The listing builds one solid part. Answer for the finished solid, in the listing's coordinates (mm). A direction names the side the tool comes from. Round coordinates to 2 decimals unless told otherwise and drop trailing zeros. Loops run counter-clockwise (first coordinate to the right, second up) from the corner with the lowest first, then second, coordinate; pieces in that order, holes last. Notation, with made-up numbers: (72, -27) -> (119, -27) arc R12 ccw to (119, -15) -> close; hole circle Ø6 at (73, 61). An arc over 180 degrees is marked (long way). One line per question, with ' | ' between items.
Autodesk Inventor part; units mm, degrees
ref_plane "YZ Plane" through (0, 0, 0) normal (1, 0, 0) x (0, 1, 0)
ref_plane "XZ Plane" through (0, 0, 0) normal (0, 1, 0) x (-1, 0, 0)
ref_plane "XY Plane" through (0, 0, 0) normal (0, 0, 1) x (1, 0, 0)
sketch "Boceto1" plane through (0, 0, 0) normal (0, 1, 0) x (-1, 0, 0)
  circle A0 centre (0, 0) radius 19.7
  circle A1 centre (0, 0) radius 22.7
  dimension "d0" = 39.4
  dimension "d1" = 45.4
extrude "Extrusión1" add sketch "Boceto1" along normal blind 40
sketch "Boceto2" plane through (0, 0, 0) normal (0, -1, 0) x (1, 0, 0)
  circle A0 centre (0, 0) radius 22.7
  circle A1 centre (0, 0) radius 19.7
extrude "Extrusión2" add sketch "Boceto2" along normal blind 3 contours A0 | A1
sketch "Boceto3" plane through (0, -3, 0) normal (0, -1, 0) x (1, 0, 0)
  circle A0 centre (0, 0) radius 10.2
  circle A1 centre (0, 0) radius 13.2
  dimension "d6" = 20.4
  dimension "d7" = 26.4
extrude "Extrusión3" add sketch "Boceto3" along normal blind 20
chamfer "Chaflán1" distance 20 angle 3 1 edges at (-13.2, -23, 0) measured on face at (13.0291, -16.3333, -2.1174)
fillet "Empalme1" radius 10 2 edges at (-13.2, -3.0001, 0) (-13.2, -3, 0)
sketch "Boceto4" plane through (0, -3, 0) normal (0, -1, 0) x (1, 0, 0)
  circle A0 centre (0, 0) radius 10.2
hole "Agujero1" at (0, -3, 0) direction (0, 1, 0) diameter 20.4 end through all
sketch "Boceto5" plane through (0, 0, 0) normal (1, 0, 0) x (0, 1, 0)
  line L0 (-23, -12.1518) -> (-23, 12.1518)
  line L1 (-12.4766, -12.7034) -> (-12.4766, 12.7034)
  line L2 (-12.4766, -12.7034) -> (-12.4766, 12.7034)
  line L3 (-3, 22.6896) -> (-3, -22.6896)
  line L4 (-23, -10.2) -> (-23, 10.2)
  line L5 (-23, 0) -> (-3, 0)
  line L6 (-3, 22.7) -> (-3, -22.7)
  line L7 (-23, 0) -> (-16.3333, 0)
  line L8 (-16.3333, 0) -> (-9.6667, 0)
  circle A0 centre (-16.3333, 0) radius 2.25
  circle A1 centre (-9.6667, 0) radius 2.25
  point P0 (0, 0)
  dimension "d21" = 6.6667
  dimension "d22" = 6.6667
  dimension "d23" = 4.5
  dimension "d24" = 4.5
hole "Agujero2" at (0, -16.3333, 0) at (0, -9.6667, 0) direction (-1, 0, 0) diameter 4.5 end through all
sketch "Boceto6" plane through (0, 0, 0) normal (0, 1, 0) x (1, 0, 0)
  circle A0 centre (0, 0) radius 25.5
  circle A1 centre (0, 0) radius 22.7
  circle A2 centre (0, 0) radius 19.7
  dimension "d32" = 51
extrude "Extrusión4" add sketch "Boceto6" against normal blind 3 contours A0
properties part number "SoporteBombilla"
Q1. For faces 4 (the face through (-5.5, -1.5, 24.9)), 5 (the face through (8, 0, -8)), 6 (the face through (-23, -3, 2)), 7 (the face through (-11.71, -7.47, 0.49)), determine the directions among +Z, -Z, +X, -X, +Y, -Y from which every point of the face is accessible in a straight line to the end or side of a thin tool.
Numbers:
face 4: +Y, -Y | face 5: +Y | face 6: -Y | face 7: -X
Q2. Find the intervals of material crossed by line 1 (Y direction, x = -12.5, z = 0); line 2 (Z direction, x = 0, y = 32.5); line 3 (X direction, y = 25, z = -13.5), in increasing order. Write a range as from..to.
Numbers:
line 1: -14.08..-11.92, -7.42..0 | line 2: -22.7..-19.7, 19.7..22.7 | line 3: -18.25..-14.35, 14.35..18.25
Q3. A cutting plane is placed at A-A on y = -2. Give the vertices of the cut face in (x, z), plus the area to 3 significant figures.
Numbers:
outline: circle Ø51 at (0, 0); hole circle Ø20.4 at (0, 0) | area: 1,720 mm^2
Q4. Given pin 1 Ø1.5 at (x, z) = (10, 12) entering from -Y; pin 2 Ø3 at (x, y) = (1, -11) entering from -Z; pin 3 Ø1 at (y, z) = (30, -1) entering from -X, each flat-ended and moving along its own axis, determine where each tip first touches the part or whether it passes through.
Numbers:
pin 1: y = -6.77 | pin 2: z = -13.29 | pin 3: x = -22.69
Q5. For a pull along Z with two mould halves and no side action, classify faces 1 (the face through (-20.97, 19.72, 8.69)), 2 (the face through (-3, -23, 10)), 3 (the face through (-11.302, -14.137, 0.488)) as pulls with the +Z half, pulls with the -Z half, needs draft (parallel to the pull), parting line crosses it, or undercut.
Numbers:
face 1: parting line crosses it | face 2: needs draft | face 3: undercut
Q6. A cutting plane is placed at B-B on y = 25. Give the vertices of the cut face in (x, z).
Numbers:
outline: circle Ø45.4 at (0, 0); hole circle Ø39.4 at (0, 0)
